Work out the finished part from the listing and answer in its coordinate system (mm). A direction names the side the tool comes from. Round coordinates to 2 decimals unless told otherwise and drop trailing zeros. Order: outer loops, then holes, each group sorted by start corner. A loop starts at its lowest first (then second) coordinate and runs counter-clockwise, first axis right, second up. Notation, with made-up numbers: M 32.25,-13.5 L 85.25,-13.5 A20 ccw 85.25,-1.5 Z; hole C -5,1 d10. An arc over 180 degrees is marked long. Return JSON: item names as keys, results as strings.
Autodesk Inventor part; units mm, degrees
ref_plane "YZ Plane" through (0, 0, 0) normal (1, 0, 0) x (0, 1, 0)
ref_plane "XZ Plane" through (0, 0, 0) normal (0, 1, 0) x (-1, 0, 0)
ref_plane "XY Plane" through (0, 0, 0) normal (0, 0, 1) x (1, 0, 0)
sketch "Skizze1" plane through (0, 0, 0) normal (0, 0, 1) x (1, 0, 0)
  line L0 (0, 0) -> (0, -20)
  line L1 (0, -20) -> (-16, -20)
  line L2 (-16, -20) -> (-16, -19)
  line L3 (-16, -19) -> (-24, -19)
  line L4 (-24, -19) -> (-24, 0)
  line L5 (-24, 0) -> (0, 0)
  dimension "d0" = 20
  dimension "d1" = 16
  dimension "d2" = 1
  dimension "d3" = 8
extrude "Main Body" add sketch "Skizze1" along normal blind 11.5
sketch "Skizze2" plane through (-24, 0, 0) normal (0, 1, 0) x (1, 0, 0)
  arc A0 (5.042, -4.5) -> (5.042, -3.5) centre (8, -4) ccw
  line L0 (0, 0) -> (0, -11.5)
  line L1 (24, -11.5) -> (0, -11.5)
  line L2 (5.042, -3.5) -> (0, -3.5)
  line L3 (5.042, -4.5) -> (0, -4.5)
  line L4 (0, -3.5) -> (0, -4.5)
  circle A1 centre (15.5, -4.5) radius 3
  circle A2 centre (21.2, -5.75) radius 1.55
  line L5 (0, 0) -> (24, 0)
  dimension "d6" = 8
  dimension "d7" = 3
  dimension "d9" = 1
  dimension "d10" = 0.5
  dimension "d11" = 6
  dimension "d13" = 15.5
  dimension "d14" = 3.1
  dimension "d15" = 21.2
  dimension "d19" = 4
  dimension "d20" = 4.5
  dimension "d21" = 5.75
extrude "Insert Holes" cut sketch "Skizze2" against normal through all
sketch "Skizze3" plane through (-16, -20, 0) normal (0, -1, 0) x (1, 0, 0)
  circle A0 centre (13.2, 5.75) radius 1.55
  line L0 (13.2, 7.3) -> (16, 7.3)
  line L1 (13.2, 4.2) -> (16, 4.2)
  line L2 (16, 0) -> (16, 11.5)
  line L3 (16, 4.2) -> (16, 7.3)
  line L4 (13.2, 7.3) -> (13.2, 4.2)
extrude "Cable Opening" cut sketch "Skizze3" against normal blind 4 contours A0 L0 L2 L1
fillet "Rundung1" radius 1 6 edges at (-16, -19, 9.25) (-16, -19, 0.5) (0, -18, 7.3) (0, -18, 4.2) (-16, -20, 9.25) (-16, -20, 0.5)
sketch "Skizze4" plane through (0, 0, 0) normal (0, 0, -1) x (-1, 0, 0)
  circle A0 centre (21.5, -15) radius 1.5
  circle A1 centre (21.5, -5.5) radius 1.5
  line L0 (24, -19) -> (24, 0)
  line L1 (24, 0) -> (0, 0)
  dimension "d25" = 3
  dimension "d26" = 3
  dimension "d27" = 2.5
  dimension "d28" = 2.5
  dimension "d29" = 5.5
  dimension "d30" = 15
extrude "Cartridge clamping holes" cut sketch "Skizze4" against normal through all
sketch "Skizze5" plane through (0, 0, 0) normal (0, 0, -1) x (-1, 0, 0)
  circle A0 centre (2.8, -10) radius 1.5
  line L0 (24, -19) -> (24, 0)
  line L1 (24, 0) -> (0, 0)
  dimension "d33" = 3
  dimension "d34" = 21.2
  dimension "d35" = 10
extrude "PT100 clamping holes" cut sketch "Skizze5" against normal up to next
chamfer "Fase1" distance 0.5 angle 45 24 edges at (0, -10, 11.5) (-7.6338, -20, 11.5) (-15.7677, -19.866, 11.5) (-20.4995, -19, 11.5) (-7.6338, -20, 0) (-15.7677, -19.866, 0) (-20.4995, -19, 0) (0, -10, 0) (0, 0, 5.75) (-12, 0, 11.5) (-24, -19, 8) (-24, -9.5, 11.5) (-24, -19, 1.75) (0, -20, 9.9) (-0.2929, -20, 7.5929) (-1.9, -20, 7.3) (-4.35, -20, 5.75) (-1.9, -20, 4.2) (-0.2929, -20, 3.9071) (0, -20, 1.6) (-12, 0, 0) (-24, -9.5, 0) (-24, 0, 1.75) (-24, 0, 8)
thread "Gewinde1"
thread "Gewinde2"
thread "Gewinde3"
thread "Gewinde4"
properties part number "E3D-v6 Volcano Heater Block" material "Aluminium 6061"
Item 1: Find section D-D (x = -21.5). Determine the outline of the cut face in (y, z).
Output:
{"outline": "M -19,0.5 L -18.5,0 L -16.5,0 L -16.5,3.5 L -19,3.5 Z; M -19,4.5 L -16.5,4.5 L -16.5,11.5 L -18.5,11.5 L -19,11 Z; M -13.5,0 L -7,0 L -7,3.5 L -13.5,3.5 Z; M -13.5,4.5 L -7,4.5 L -7,11.5 L -13.5,11.5 Z; M -4,0 L -0.5,0 L 0,0.5 L 0,3.5 L -4,3.5 Z; M -4,4.5 L 0,4.5 L 0,11 L -0.5,11.5 L -4,11.5 Z"}
Item 2: Find section A-A (y = -15). Determine the outline of the cut face in (x, z), plus the area to 3 significant figures.
Output:
{"outline": "M -24,0.5 L -23.5,0 L -23,0 L -23,3.5 L -24,3.5 Z; M -24,4.5 L -23,4.5 L -23,11.5 L -23.5,11.5 L -24,11 Z; M -20,0 L -0.5,0 L 0,0.5 L 0,11 L -0.5,11.5 L -20,11.5 L -20,4.5 L -18.96,4.5 A3 cw long -18.96,3.5 L -20,3.5 Z; hole C -8.5,4.5 d6; hole C -2.8,5.75 d3.1", "area": "175 mm^2"}
Item 3: Which of the six approach directions +Z, -Z, +X, -X, +Y, -Y give full straight-line access (tool end or side, diameter ignored) to faces 1 (the flat face through (-1, -16, 6)), 2 (the flat face through (-21, -9, 4.5)), 3 (the flat face through (-20, -19, 8))?
Output:
{"face 1": "+X, -Y", "face 2": "-X, +Y, -Y", "face 3": "+Z, -Z, -X, -Y"}
Item 4: The mould has two halves that part along Y. Classify faces 4 (the flat face through (-21, -9, 3.5)), 5 (the cylindrical face through (-20, -5.43, 1.73)), 6 (the cylindrical face through (-16.49, -19.14, 8.94)): pulls with the +Y half, pulls with the -Y half, needs draft (parallel to the pull), parting line crosses it, or undercut.
Output:
{"face 4": "needs draft", "face 5": "undercut", "face 6": "pulls with the -Y half"}
Item 5: Each of these flat-tipped pins is pushed along its axis until it touches: pin 1 (0.9 mm diameter, centred on x = -22, z = 1.5, fed in from -Y); pin 2 (2.5 mm diameter, centred on x = -2.8, z = 5.75, fed in from +Y); pin 3 (1.4 mm diameter, centred on x = -1.5, z = 5, fed in from -Y). Where does it stop, or does it pass through?
Output:
{"pin 1": "stops at y = -19", "pin 2": "passes through", "pin 3": "stops at y = -16"}
Item 6: Find section B-B (x = -8.5). Determine the outline of the cut face in (y, z).
Output:
{"outline": "M -20,0.5 L -19.5,0 L -0.5,0 L 0,0.5 L 0,1.5 L -20,1.5 Z; M -20,7.5 L 0,7.5 L 0,11 L -0.5,11.5 L -19.5,11.5 L -20,11 Z"}
Item 7: Find section C-C (z = 2). Determine the outline of the cut face in (x, y), plus the area to 3 significant figures.
Output:
{"outline": "M -24,-18.5 L -23.5,-19 L -18.24,-19 L -18.24,0 L -23.5,0 L -24,-0.5 Z; M -13.76,-20 L -10.16,-20 L -10.16,0 L -13.76,0 Z; M -6.84,-20 L -0.5,-20 L 0,-19.5 L 0,-0.5 L -0.5,0 L -6.84,0 Z; hole C -21.5,-15 d3; hole C -21.5,-5.5 d3; hole C -2.8,-10 d3", "area": "297 mm^2"}
Item 8: Consider line 1 along Y through (x, z) = (-21.5, 2.55); line 2 along Z through (x, y) = (-22.5, -8.75); line 3 along Z through (x, y) = (-16, -12.25). Determine where each line is inside the solid, lowest interval first. Write a range as [from, to].
Output:
{"line 1": "y = [-19, -16.5], [-13.5, -7], [-4, 0]", "line 2": "z = [0, 3.5], [4.5, 11.5]", "line 3": "z = [0, 1], [7, 11.5]"}
